Work out the finished part from the listing and answer in its coordinate system (mm). A direction names the side the tool comes from. Give positions to 0.01 mm unless a question says otherwise; leave off trailing zeros. Loops run counter-clockwise (first coordinate to the right, second up) from the corner with the lowest first, then second, coordinate; pieces in that order, holes last. Notation, with made-up numbers: M -10,20.25 L 25,20.25 A16 cw 25,35.25 Z; hole C 26.25,85.25 d5. An arc over 180 degrees is marked long. Use a Markdown table: item, result.
```python
from build123d import *

# Parameters (mm, degrees)
CROQUIS1_W              = 77.1
CROQUIS1_H              = 42.7
SALIENTE_EXTRUIR1_DEPTH = 1.6
CROQUIS2_W              = 60.3
CROQUIS2_H              = 42.2
SALIENTE_EXTRUIR2_DEPTH = 3.7
CORTAR_EXTRUIR1_REACH   = 3.6
CROQUIS3_R              = 0.5


with BuildPart() as part:
    # Croquis1 → Saliente-Extruir1 (new body)
    with BuildSketch(Plane(origin=(0, 0, 0), x_dir=(1, 0, 0), z_dir=(0, 1, 0))):
        Rectangle(CROQUIS1_W, CROQUIS1_H)
    extrude(amount=SALIENTE_EXTRUIR1_DEPTH)

    # Croquis2 → Saliente-Extruir2 (add)
    with BuildSketch(Plane(origin=(0, 1.6, 0), x_dir=(1, 0, 0), z_dir=(0, 1, 0))):
        with Locations((-1.5, 0)):
            Rectangle(CROQUIS2_W, CROQUIS2_H)
    extrude(amount=SALIENTE_EXTRUIR2_DEPTH)

    # Croquis3 → Cortar-Extruir1 (cut, up to next)
    with BuildSketch(Plane(origin=(0, 1.6, 0), x_dir=(1, 0, 0), z_dir=(0, 1, 0)), mode=Mode.PRIVATE) as cortar_extruir1_sk1:
        with Locations((37.05, -15.923235508)):
            Circle(CROQUIS3_R)
    cortar_extruir1_tool1 = extrude(cortar_extruir1_sk1.sketch, amount=-CORTAR_EXTRUIR1_REACH, mode=Mode.PRIVATE) & part.part
    add(cortar_extruir1_tool1.solids().sort_by_distance((37.05, 1.6, 15.923236))[0], mode=Mode.SUBTRACT)
    # Croquis3 → Cortar-Extruir1 (cut, up to next)
    with BuildSketch(Plane(origin=(0, 1.6, 0), x_dir=(1, 0, 0), z_dir=(0, 1, 0)), mode=Mode.PRIVATE) as cortar_extruir1_sk2:
        with Locations((37.05, -13.383235508)):
            Circle(CROQUIS3_R)
    cortar_extruir1_tool2 = extrude(cortar_extruir1_sk2.sketch, amount=-CORTAR_EXTRUIR1_REACH, mode=Mode.PRIVATE) & part.part
    add(cortar_extruir1_tool2.solids().sort_by_distance((37.05, 1.6, 13.383236))[0], mode=Mode.SUBTRACT)
    # Croquis3 → Cortar-Extruir1 (cut, up to next)
    with BuildSketch(Plane(origin=(0, 1.6, 0), x_dir=(1, 0, 0), z_dir=(0, 1, 0)), mode=Mode.PRIVATE) as cortar_extruir1_sk3:
        with Locations((37.05, -10.843235508)):
            Circle(CROQUIS3_R)
    cortar_extruir1_tool3 = extrude(cortar_extruir1_sk3.sketch, amount=-CORTAR_EXTRUIR1_REACH, mode=Mode.PRIVATE) & part.part
    add(cortar_extruir1_tool3.solids().sort_by_distance((37.05, 1.6, 10.843236))[0], mode=Mode.SUBTRACT)
    # Croquis3 → Cortar-Extruir1 (cut, up to next)
    with BuildSketch(Plane(origin=(0, 1.6, 0), x_dir=(1, 0, 0), z_dir=(0, 1, 0)), mode=Mode.PRIVATE) as cortar_extruir1_sk4:
        with Locations((37.05, -8.303235508)):
            Circle(CROQUIS3_R)
    cortar_extruir1_tool4 = extrude(cortar_extruir1_sk4.sketch, amount=-CORTAR_EXTRUIR1_REACH, mode=Mode.PRIVATE) & part.part
    add(cortar_extruir1_tool4.solids().sort_by_distance((37.05, 1.6, 8.303236))[0], mode=Mode.SUBTRACT)
    # Croquis3 → Cortar-Extruir1 (cut, up to next)
    with BuildSketch(Plane(origin=(0, 1.6, 0), x_dir=(1, 0, 0), z_dir=(0, 1, 0)), mode=Mode.PRIVATE) as cortar_extruir1_sk5:
        with Locations((37.05, -5.763235508)):
            Circle(CROQUIS3_R)
    cortar_extruir1_tool5 = extrude(cortar_extruir1_sk5.sketch, amount=-CORTAR_EXTRUIR1_REACH, mode=Mode.PRIVATE) & part.part
    add(cortar_extruir1_tool5.solids().sort_by_distance((37.05, 1.6, 5.763236))[0], mode=Mode.SUBTRACT)
    # Croquis3 → Cortar-Extruir1 (cut, up to next)
    with BuildSketch(Plane(origin=(0, 1.6, 0), x_dir=(1, 0, 0), z_dir=(0, 1, 0)), mode=Mode.PRIVATE) as cortar_extruir1_sk6:
        with Locations((37.05, -3.223235508)):
            Circle(CROQUIS3_R)
    cortar_extruir1_tool6 = extrude(cortar_extruir1_sk6.sketch, amount=-CORTAR_EXTRUIR1_REACH, mode=Mode.PRIVATE) & part.part
    add(cortar_extruir1_tool6.solids().sort_by_distance((37.05, 1.6, 3.223236))[0], mode=Mode.SUBTRACT)
    # Croquis3 → Cortar-Extruir1 (cut, up to next)
    with BuildSketch(Plane(origin=(0, 1.6, 0), x_dir=(1, 0, 0), z_dir=(0, 1, 0)), mode=Mode.PRIVATE) as cortar_extruir1_sk7:
        with Locations((37.05, -0.683235508)):
            Circle(CROQUIS3_R)
    cortar_extruir1_tool7 = extrude(cortar_extruir1_sk7.sketch, amount=-CORTAR_EXTRUIR1_REACH, mode=Mode.PRIVATE) & part.part
    add(cortar_extruir1_tool7.solids().sort_by_distance((37.05, 1.6, 0.683236))[0], mode=Mode.SUBTRACT)
    # Croquis3 → Cortar-Extruir1 (cut, up to next)
    with BuildSketch(Plane(origin=(0, 1.6, 0), x_dir=(1, 0, 0), z_dir=(0, 1, 0)), mode=Mode.PRIVATE) as cortar_extruir1_sk8:
        with Locations((37.05, 1.856764492)):
            Circle(CROQUIS3_R)
    cortar_extruir1_tool8 = extrude(cortar_extruir1_sk8.sketch, amount=-CORTAR_EXTRUIR1_REACH, mode=Mode.PRIVATE) & part.part
    add(cortar_extruir1_tool8.solids().sort_by_distance((37.05, 1.6, -1.856764))[0], mode=Mode.SUBTRACT)
    # Croquis3 → Cortar-Extruir1 (cut, up to next)
    with BuildSketch(Plane(origin=(0, 1.6, 0), x_dir=(1, 0, 0), z_dir=(0, 1, 0)), mode=Mode.PRIVATE) as cortar_extruir1_sk9:
        with Locations((37.05, 4.396764492)):
            Circle(CROQUIS3_R)
    cortar_extruir1_tool9 = extrude(cortar_extruir1_sk9.sketch, amount=-CORTAR_EXTRUIR1_REACH, mode=Mode.PRIVATE) & part.part
    add(cortar_extruir1_tool9.solids().sort_by_distance((37.05, 1.6, -4.396764))[0], mode=Mode.SUBTRACT)
    # Croquis3 → Cortar-Extruir1 (cut, up to next)
    with BuildSketch(Plane(origin=(0, 1.6, 0), x_dir=(1, 0, 0), z_dir=(0, 1, 0)), mode=Mode.PRIVATE) as cortar_extruir1_sk10:
        with Locations((37.05, 6.936764492)):
            Circle(CROQUIS3_R)
    cortar_extruir1_tool10 = extrude(cortar_extruir1_sk10.sketch, amount=-CORTAR_EXTRUIR1_REACH, mode=Mode.PRIVATE) & part.part
    add(cortar_extruir1_tool10.solids().sort_by_distance((37.05, 1.6, -6.936764))[0], mode=Mode.SUBTRACT)
    # Croquis3 → Cortar-Extruir1 (cut, up to next)
    with BuildSketch(Plane(origin=(0, 1.6, 0), x_dir=(1, 0, 0), z_dir=(0, 1, 0)), mode=Mode.PRIVATE) as cortar_extruir1_sk11:
        with Locations((37.05, 9.476764492)):
            Circle(CROQUIS3_R)
    cortar_extruir1_tool11 = extrude(cortar_extruir1_sk11.sketch, amount=-CORTAR_EXTRUIR1_REACH, mode=Mode.PRIVATE) & part.part
    add(cortar_extruir1_tool11.solids().sort_by_distance((37.05, 1.6, -9.476764))[0], mode=Mode.SUBTRACT)
    # Croquis3 → Cortar-Extruir1 (cut, up to next)
    with BuildSketch(Plane(origin=(0, 1.6, 0), x_dir=(1, 0, 0), z_dir=(0, 1, 0)), mode=Mode.PRIVATE) as cortar_extruir1_sk12:
        with Locations((37.05, 12.016764492)):
            Circle(CROQUIS3_R)
    cortar_extruir1_tool12 = extrude(cortar_extruir1_sk12.sketch, amount=-CORTAR_EXTRUIR1_REACH, mode=Mode.PRIVATE) & part.part
    add(cortar_extruir1_tool12.solids().sort_by_distance((37.05, 1.6, -12.016764))[0], mode=Mode.SUBTRACT)
    # Croquis3 → Cortar-Extruir1 (cut, up to next)
    with BuildSketch(Plane(origin=(0, 1.6, 0), x_dir=(1, 0, 0), z_dir=(0, 1, 0)), mode=Mode.PRIVATE) as cortar_extruir1_sk13:
        with Locations((37.05, 14.556764492)):
            Circle(CROQUIS3_R)
    cortar_extruir1_tool13 = extrude(cortar_extruir1_sk13.sketch, amount=-CORTAR_EXTRUIR1_REACH, mode=Mode.PRIVATE) & part.part
    add(cortar_extruir1_tool13.solids().sort_by_distance((37.05, 1.6, -14.556764))[0], mode=Mode.SUBTRACT)
    # Croquis3 → Cortar-Extruir1 (cut, up to next)
    with BuildSketch(Plane(origin=(0, 1.6, 0), x_dir=(1, 0, 0), z_dir=(0, 1, 0)), mode=Mode.PRIVATE) as cortar_extruir1_sk14:
        with Locations((37.05, 17.096764492)):
            Circle(CROQUIS3_R)
    cortar_extruir1_tool14 = extrude(cortar_extruir1_sk14.sketch, amount=-CORTAR_EXTRUIR1_REACH, mode=Mode.PRIVATE) & part.part
    add(cortar_extruir1_tool14.solids().sort_by_distance((37.05, 1.6, -17.096764))[0], mode=Mode.SUBTRACT)


solid = part.part
```
(1) A cutting plane is placed at A-A (z = 18.5). Write down the section's boundary in (x, y).
Entries:
| item | result |
|---|---|
| outline | M -38.55,0 L 38.55,0 L 38.55,1.6 L 28.65,1.6 L 28.65,5.3 L -31.65,5.3 L -31.65,1.6 L -38.55,1.6 Z |
(2) A cutting plane is placed at B-B (y = 3). Write down the section's boundary in (x, z), and give its area (3 significant figures).
Entries:
| item | result |
|---|---|
| outline | M -31.65,-21.1 L 28.65,-21.1 L 28.65,21.1 L -31.65,21.1 Z |
| area | 2,540 mm² |
(3) Given P1, Ø1.1, axis at y = 4, z = 6.5, coming from the +X side; P2, Ø1.5, axis at x = 3, z = 2.5, coming from the -Y side; P3, Ø1.9, axis at x = 12, y = 3, coming from the -Z side; P4, Ø3, axis at y = 4, z = 5.5, coming from the -X side, each flat-ended and moving along its own axis, determine where each tip first touches the part or whether it passes through.
Entries:
| item | result |
|---|---|
| P1 | stops at x = 28.65 |
| P2 | stops at y = 0 |
| P3 | stops at z = -21.1 |
| P4 | stops at x = -31.65 |
(4) Consider probe 1 along Z at (x, y) = (-23.5, 4.05); probe 2 along Y at (x, z) = (31.5, 2); probe 3 along X at (y, z) = (3.1, -10). Determine where each line is inside the solid, lowest interval first. Write a range as [from, to].
Entries:
| item | result |
|---|---|
| probe 1 | z = [-21.1, 21.1] |
| probe 2 | y = [0, 1.6] |
| probe 3 | x = [-31.65, 28.65] |
(5) Which of the six approach directions +Z, -Z, +X, -X, +Y, -Y give full straight-line access (tool end or side, diameter ignored) to faces 1 (the flat face through (28.65, 3, 0)), 2 (the flat face through (-2, 3, 21.1)), 3 (the flat face through (-31.65, 3, 0)), 4 (the flat face through (-38.55, 1, 0)), 5 (the flat face through (-2, 3, -21.1))?
Entries:
| item | result |
|---|---|
| face 1 | +Z, -Z, +X, +Y |
| face 2 | +Z, +X, -X, +Y |
| face 3 | +Z, -Z, -X, +Y |
| face 4 | +Z, -Z, -X, +Y, -Y |
| face 5 | -Z, +X, -X, +Y |
